```python
from build123d import *

# Parameters (mm, degrees)
F0_R     = 17.4625
F0_R_2   = 12.7
F1_DEPTH = 5.08
F0_R_3   = 1.5875
F2_R     = 17.4625
F3_DEPTH = 9.525
F4_DEPTH = 9.525
F5_DEPTH = 6.35
F6_W     = 9.652
F6_H     = 9.652
F7_DEPTH = 12.7
F8_R     = 0.762
F9_SIZE  = 0.508


with BuildPart() as f1:
    # F0 (on Front) → F1 (new body)
    with BuildSketch(Plane.XZ):
        Circle(F0_R)
        Circle(F0_R_2, mode=Mode.SUBTRACT)
    extrude(amount=F1_DEPTH)



with BuildPart() as f1b:
    # F0 (on Front) → F1, piece 2 (new body)
    with BuildSketch(Plane.XZ):
        with Locations((0, 6.35)):
            Circle(F0_R_3)
    extrude(amount=F1_DEPTH)


with BuildPart() as f1c:
    # F0 (on Front) → F1, piece 3 (new body)
    with BuildSketch(Plane.XZ):
        with Locations((6.35, 0)):
            Circle(F0_R_3)
    extrude(amount=F1_DEPTH)


with BuildPart() as f1d:
    # F0 (on Front) → F1, piece 4 (new body)
    with BuildSketch(Plane.XZ):
        with Locations((0, -6.35)):
            Circle(F0_R_3)
    extrude(amount=F1_DEPTH)


with BuildPart() as f1e:
    # F0 (on Front) → F1, piece 5 (new body)
    with BuildSketch(Plane.XZ):
        with Locations((-6.35, 0)):
            Circle(F0_R_3)
    extrude(amount=F1_DEPTH)


with BuildPart() as f1_1:
    add(f1.part)

    add(f1b.part)  # F3 merges F1b

    add(f1c.part)  # F3 merges F1c

    add(f1d.part)  # F3 merges F1d

    add(f1e.part)  # F3 merges F1e
    # F2 (on face) → F3 (join)
    with BuildSketch(Plane(origin=(0, 0, 0), x_dir=(-1, 0, 0), z_dir=(0, 1, 0))):
        Circle(F2_R)
    extrude(amount=F3_DEPTH)

    # F4 (add): a face of the model
    f4_faces = [f1_1.faces().sort_by_distance(p)[0] for p in [
        (-16.9685859133, -5.08, 0),
    ]]
    extrude(f4_faces, amount=F4_DEPTH)

    # F5 (add): a face of the model
    f5_faces = [f1_1.faces().sort_by_distance(p)[0] for p in [
        (0, 9.525, 0),
    ]]
    extrude(f5_faces, amount=F5_DEPTH)

    # F6 (on face) → F7 (cut)
    with BuildSketch(Plane(origin=(0, 15.875, 0), x_dir=(-1, 0, 0), z_dir=(0, 1, 0))):
        Rectangle(F6_W, F6_H)
    extrude(amount=-F7_DEPTH, mode=Mode.SUBTRACT)

    # F8
    f8_edges = [f1_1.edges().sort_by_distance(p)[0] for p in [
        (4.826, 9.525, 4.826),
        (4.826, 9.525, -4.826),
        (-4.826, 9.525, -4.826),
        (-4.826, 9.525, 4.826),
    ]]
    fillet(f8_edges, radius=F8_R)

    # F9
    f9_edges = [f1_1.edges().sort_by_distance(p)[0] for p in [
        (0, 15.875, 4.826),
        (17.4625, 15.875, 0),
        (-17.4625, -14.605, 0),
        (-12.7, -14.605, 0),
        (-1.5875, -5.08, -6.35),
        (4.7625, -5.08, 0),
        (-1.5875, -5.08, 6.35),
        (-7.9375, -5.08, 0),
    ]]
    chamfer(f9_edges, length=F9_SIZE)


solid = f1_1.part
```
Geometry: final body of the model. Coordinates: model frame, mm. A direction names the side the tool comes from. Round coordinates to 2 decimals unless told otherwise and drop trailing zeros. Order: outer loops, then holes, each group sorted by start corner. A loop starts at its lowest first (then second) coordinate and runs counter-clockwise, first axis right, second up. Notation, with made-up numbers: M 10.5,23.5 L 54.5,23.5 A28 ccw 54.5,61.5 Z; hole C 32.5,-10.5 d10. An arc over 180 degrees is marked long. One line per item, written item: value.
(1) Cut plane D-D (y = -11.5). Return the cut outline in (x, z) (1 decimal), and give its area (3 significant figures).
Result sheet:
outline: C 0,0 d34.9; hole C 0,0 d25.4
area: 451 mm2
(2) Pull-direction query (Z, two-part tool) for faces 1 (the flat face through (-6, -5.08, 0)), 2 (the cylindrical face through (-0.34, -2.25, -7.9)); classes: pulls with the +Z half, pulls with the -Z half, needs draft (parallel to the pull), parting line crosses it, or undercut.
Result sheet:
face 1: undercut
face 2: undercut
(3) Pin query (flat end, axial travel): P1, Ø6, axis at x = 0.5, z = -1.5, coming from the -Y side; P2, Ø1.7, axis at x = 6, z = 0.5, coming from the -Y side; P3, Ø5, axis at y = 1, z = 3.5, coming from the +X side. Return the tip coordinate at first contact, or that it passes through.
Result sheet:
P1: y = 0
P2: y = -5.08
P3: x = 17.43
(4) Line query: probe 1 along Z at (x, y) = (0, -1); probe 2 along Z at (x, y) = (0, -12); probe 3 along Y at (x, z) = (0, 12.5) (3 decimals). Output: solid intervals per line, ascending. Write a range as [from, to].
Result sheet:
probe 1: [-17.46, -12.7], [-7.94, -4.76], [4.76, 7.94], [12.7, 17.46]
probe 2: [-17.46, -12.7], [12.7, 17.46]
probe 3: [0, 15.875]
(5) Reachability of faces 3 (the cylindrical face through (-4.836, -2.254, 0.477)), 4 (the flat face through (0, 9, 4.826)) from +Z, -Z, +X, -X, +Y, -Y: full face, straight path, thin tool, end or side. Return the list, or none.
Result sheet:
face 3: -Y
face 4: +Y
(6) Cut plane A-A (y = -2). Give the number of separate pieces and of enclosed holes in the cut face, and give its area (3 significant figures).
Result sheet:
separate pieces: 5
enclosed holes: 1
area: 483 mm2
